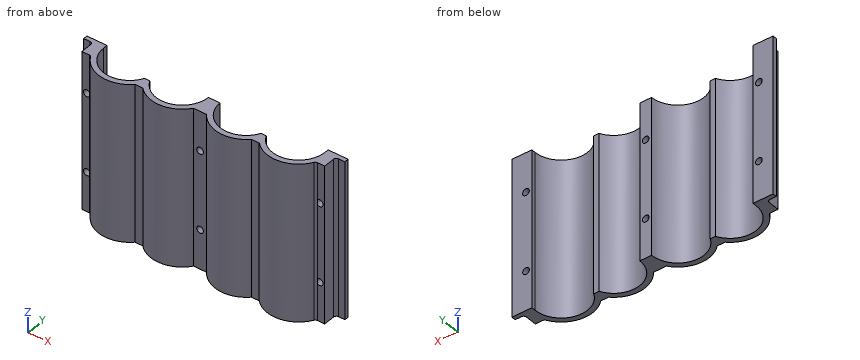
from build123d import *

# Parameters (mm, degrees)
BOSS_EXTRUDE1_DEPTH                         = 60
FILLET1_R                                   = 1
TAPPED_START                                = -7
TAPPED_HOLE_FOR_M2_5X0_45_HELICOIL1_OUTL_R  = 1.275
TAPPED_HOLE_FOR_M2_5X0_45_HELICOIL1_DEPTH   = 7
TAPPED_START_2                              = -8.6
TAPPED_HOLE_FOR_M2_5X0_45_HELICOIL1_2_OU_R  = 1.275
TAPPED_HOLE_FOR_M2_5X0_45_HELICOIL1_2_DEPTH = 1.6


# Read off the part's stored shape, not the designer's step: Tapped Hole for M2.5x0.45 Helicoil1
with BuildPart() as part:
    # Sketch1 → Boss-Extrude1 (new body)
    with BuildSketch(Plane.XY):
        with BuildLine():
            Line((0, 0), (7.65, 0))
            Line((7.65, 0), (7.65, -1.6))
            ThreePointArc((7.65, -1.6), (15.413932023, -11.346794345), (26.65, -5.958898944))
            Line((26.65, -5.958898944), (28.65, -5.958898944))
            ThreePointArc((28.65, -5.958898944), (39.886067977, -11.346794345), (47.65, -1.6))
            Line((47.65, -1.6), (52.15, -1.6))
            ThreePointArc((52.15, -1.6), (59.913932023, -11.346794345), (71.15, -5.958898944))
            Line((71.15, -5.958898944), (73.15, -5.958898944))
            ThreePointArc((73.15, -5.958898944), (84.386067977, -11.346794345), (92.15, -1.6))
            Line((92.15, -1.6), (92.15, 0))
            Line((92.15, 0), (99.8, 0))
            Line((99.8, 0), (99.8, -1.6))
            Line((99.8, -1.6), (96.3, -1.6))
            Line((96.3, -1.6), (96.3, -7))
            Line((96.3, -7), (92.86634266, -7))
            ThreePointArc((92.86634266, -7), (84.043434268, -13.449679602), (73.65, -10.070537173))
            Line((73.65, -10.070537173), (70.65, -10.070537173))
            ThreePointArc((70.65, -10.070537173), (61.186027008, -13.561218837), (52.403205655, -8.6))
            Line((52.403205655, -8.6), (47.396794345, -8.6))
            ThreePointArc((47.396794345, -8.6), (38.613972992, -13.561218837), (29.15, -10.070537173))
            Line((29.15, -10.070537173), (26.15, -10.070537173))
            ThreePointArc((26.15, -10.070537173), (15.756565732, -13.449679602), (6.93365734, -7))
            Line((6.93365734, -7), (3.5, -7))
            Line((3.5, -7), (3.5, -1.6))
            Line((3.5, -1.6), (0, -1.6))
            Line((0, -1.6), (0, 0))
        make_face()
    extrude(amount=BOSS_EXTRUDE1_DEPTH)

    # Fillet1
    fillet1_edges = [part.edges().sort_by_distance(p)[0] for p in [
        (96.3, -1.6, 30),
        (92.86634266, -7, 30),
        (6.93365734, -7, 30),
        (3.5, -1.6, 30),
    ]]
    fillet(fillet1_edges, radius=FILLET1_R)

    # Tapped Hole for M2.5x0.45 Helicoil1 outl → Tapped Hole for M2.5x0.45 Helicoil1 (cut)
    with BuildSketch(Plane(origin=(0, 0, 0), x_dir=(1, 0, 0), z_dir=(0, 1, 0)).offset(TAPPED_START)):
        with Locations((94.4, -15)):
            Circle(TAPPED_HOLE_FOR_M2_5X0_45_HELICOIL1_OUTL_R)
        with Locations((94.4, -45)):
            Circle(TAPPED_HOLE_FOR_M2_5X0_45_HELICOIL1_OUTL_R)
        with Locations((49.9, -15)):
            Circle(TAPPED_HOLE_FOR_M2_5X0_45_HELICOIL1_OUTL_R)
        with Locations((49.9, -45)):
            Circle(TAPPED_HOLE_FOR_M2_5X0_45_HELICOIL1_OUTL_R)
    tapped_hole_for_m2_5x0_45_helicoil1 = extrude(amount=TAPPED_HOLE_FOR_M2_5X0_45_HELICOIL1_DEPTH, mode=Mode.SUBTRACT)

    # Tapped Hole for M2.5x0.45 Helicoil1 2 ou → Tapped Hole for M2.5x0.45 Helicoil1 2 (cut)
    with BuildSketch(Plane(origin=(0, 0, 0), x_dir=(1, 0, 0), z_dir=(0, 1, 0)).offset(TAPPED_START_2)):
        with Locations((49.9, -15)):
            Circle(TAPPED_HOLE_FOR_M2_5X0_45_HELICOIL1_2_OU_R)
        with Locations((49.9, -45)):
            Circle(TAPPED_HOLE_FOR_M2_5X0_45_HELICOIL1_2_OU_R)
    tapped_hole_for_m2_5x0_45_helicoil1_2 = extrude(amount=TAPPED_HOLE_FOR_M2_5X0_45_HELICOIL1_2_DEPTH, mode=Mode.SUBTRACT)

    # Mirror1: Tapped Hole for M2.5x0.45 Helicoil1, Tapped Hole for M2.5x0.45 Helicoil1 2 across plane
    add(tapped_hole_for_m2_5x0_45_helicoil1.mirror(Plane.ZY.offset(-49.9)), mode=Mode.SUBTRACT)
    add(tapped_hole_for_m2_5x0_45_helicoil1_2.mirror(Plane.ZY.offset(-49.9)), mode=Mode.SUBTRACT)


solid = part.part
Can you work these out from the model? Positions are in its coordinate system, mm. Round coordinates to 2 decimals unless told otherwise and drop trailing zeros. Loops run counter-clockwise (first coordinate to the right, second up) from the corner with the lowest first, then second, coordinate; pieces in that order, holes last. Notation, with made-up numbers: (-32, 82.25) - (5, 82.25) arc R21 ccw to (5, 120.25) - close; hole circle Ø8 at (60.25, 34.25). An arc over 180 degrees is marked (long way). Write item = value, one per line. Start each with the question number.
(1) If I drill on probe 1 along Z at (x, y) = (49.9, -4.75) (3 decimals); probe 2 along X at (y, z) = (-3.5, 36.5); probe 3 along X at (y, z) = (-11.75, 53), over which ranges is the centre line in solid material (lowest first)? Write a range as [from, to].
(2) If we section it at C-C (x = 15.5): Please give me the cut outline in (y, z).
(3) For P1, Ø0.9, axis at x = 95.5, z = 22, coming from the -Y side; P2, Ø8, axis at x = 33, z = 12, coming from the +Y side; P3, Ø4, axis at x = 54, z = 14.5, coming from the +Y side, each with a flat end and sliding along its axis, tell me the tip position at first contact or that it passes through.
(4) If we section it at A-A (x = 49.9): Please give me the cut outline in (y, z) (3 decimals).
(5) If we section it at D-D (x = 88): Please give me the cut outline in (y, z), and give its area (3 significant figures).
Ans:
q1.probe_1 = [0, 13.725], [16.275, 43.725], [46.275, 60]
q1.probe_2 = [3.5, 7.83], [47.47, 52.33], [91.97, 96.3]
q1.probe_3 = [11.25, 24.05], [31.25, 44.05], [55.75, 68.55], [75.75, 88.55]
q2.outline = (-13.41, 0) - (-11.37, 0) - (-11.37, 60) - (-13.41, 60) - close
q3.P1 = -7
q3.P2 = -6.62
q3.P3 = -1.6
q4.outline = (-8.6, 0) - (-1.6, 0) - (-1.6, 13.725) - (-8.6, 13.725) - close; (-8.6, 16.275) - (-1.6, 16.275) - (-1.6, 43.725) - (-8.6, 43.725) - close; (-8.6, 46.275) - (-1.6, 46.275) - (-1.6, 60) - (-8.6, 60) - close
q5.outline = (-12.08, 0) - (-9.71, 0) - (-9.71, 60) - (-12.08, 60) - close
q5.area = 142 mm²
